Geometry: see drawing. Coordinates: mm, zero at the bounding-box minimum. Give positions to 0.01 mm unless a question says otherwise; leave off trailing zeros. Loops run counter-clockwise (first coordinate to the right, second up) from the corner with the lowest first, then second, coordinate; pieces in that order, holes last. Notation, with made-up numbers: M 21.5,-12.75 L 49.5,-12.75 A22 ccw 49.5,20.25 Z; hole C -12.5,3.25 d2. An arc over 180 degrees is marked long. Use a Markdown table: item, result. Add a question column.
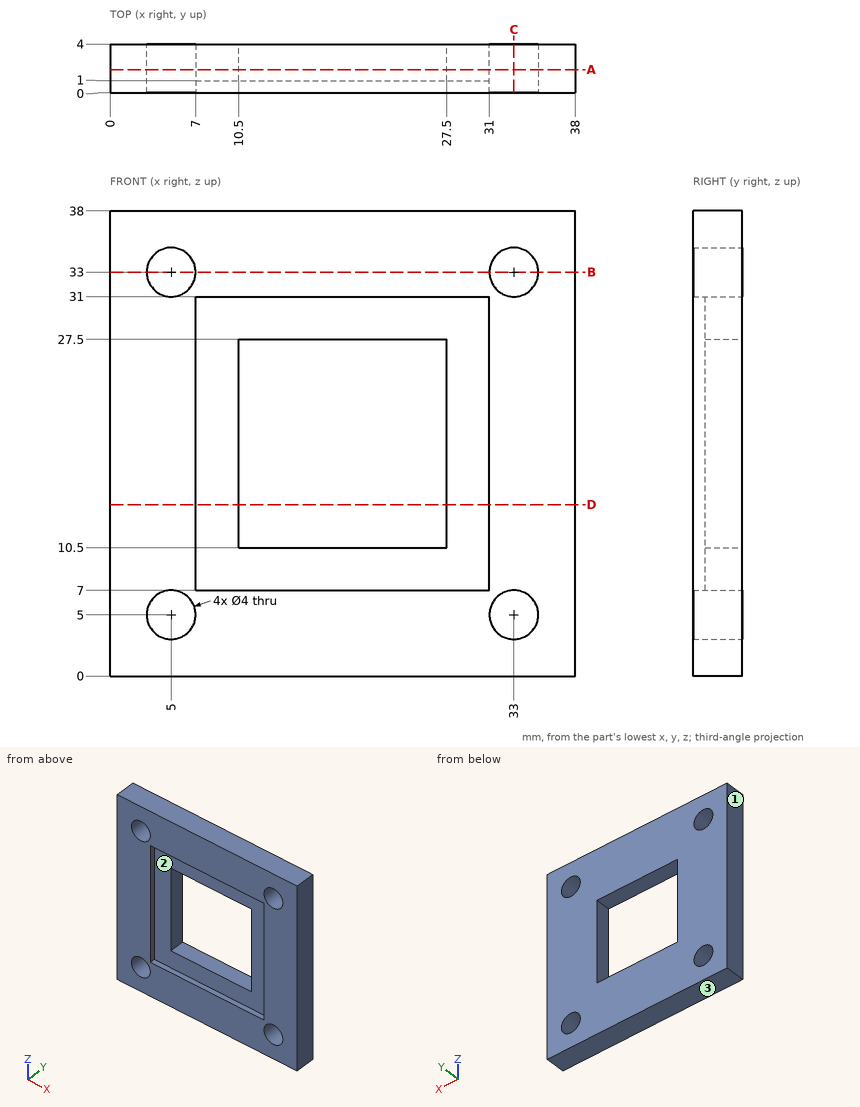
1) Pull-direction query (X, two-part tool) for the marked faces 1, 2 and 3; classes: pulls with the +X half, pulls with the -X half, needs draft (parallel to the pull), parting line crosses it, or undercut.
2) Section query B-B, the plane z = 33. Return the cut outline in (x, y).
3) Section query D-D, the plane z = 14. Return the cut outline in (x, y), and give its area (3 significant figures).
4) Section query A-A, the plane y = 1.9. Return the cut outline in (x, z), and give its area (3 significant figures).
5) Ray query, line 1 (Z direction, x = 12, y = 0.8); line 2 (X direction, y = 2.95, z = 21). Return the intervals inside material, ascending. Write a range as [from, to].
6) Section query C-C, the plane x = 33. Return the cut outline in (y, z), and give its area (3 significant figures).
7) Contact query for a flat-ended pin moving along its axis: P1, Ø12, axis at x = 22, z = 19.5, coming from the -Y side. Output: stop coordinate, or through.
Entries:
| question | item | result |
|---|---|---|
| 1 | face 1 | pulls with the -X half |
| 1 | face 2 | undercut |
| 1 | face 3 | needs draft |
| 2 | outline | M 0,0 L 3,0 L 3,4 L 0,4 Z; M 7,0 L 31,0 L 31,4 L 7,4 Z; M 35,0 L 38,0 L 38,4 L 35,4 Z |
| 3 | outline | M 0,0 L 7,0 L 7,1 L 10.5,1 L 10.5,4 L 0,4 Z; M 27.5,1 L 31,1 L 31,0 L 38,0 L 38,4 L 27.5,4 Z |
| 3 | area | 77.0 mm² |
| 4 | outline | M 0,0 L 38,0 L 38,38 L 0,38 Z; hole C 5,5 d4; hole C 5,33 d4; hole M 10.5,10.5 L 27.5,10.5 L 27.5,27.5 L 10.5,27.5 Z; hole C 33,5 d4; hole C 33,33 d4 |
| 4 | area | 1,100 mm² |
| 5 | line 1 | z = [0, 7], [31, 38] |
| 5 | line 2 | x = [0, 10.5], [27.5, 38] |
| 6 | outline | M 0,0 L 4,0 L 4,3 L 0,3 Z; M 0,7 L 4,7 L 4,31 L 0,31 Z; M 0,35 L 4,35 L 4,38 L 0,38 Z |
| 6 | area | 120 mm² |
| 7 | P1 | stops at y = 1 |
